Model file for the job. Use its own axes, mm. Face numbers are marked on the shaded views. A direction names the side the tool comes from. Give positions to 0.01 mm unless a question says otherwise; leave off trailing zeros. Loops run counter-clockwise (first coordinate to the right, second up) from the corner with the lowest first, then second, coordinate; pieces in that order, holes last. Notation, with made-up numbers: M -23,-33.5 L 8,-33.5 A12 ccw 8,-10.5 Z; hole C 42,46.25 d3. An arc over 180 degrees is marked long. Answer in a Markdown table with one row per item.
```python
from build123d import *

# Parameters (mm, degrees)
F1_DEPTH = 2.5
F3_DEPTH = 1
F4_DEPTH = 2.5
F5_R     = 5
F6_DEPTH = 2.5


with BuildPart() as f1:
    # F0 (on Top) → F1 (new body)
    with BuildSketch(Plane.XY):
        Polygon((24.5, 28.75), (-24.5, 28.75), (-38, 16), (0, -28), (38, 16), align=None)
    extrude(amount=F1_DEPTH)

    # F2 (on face) → F3 (join)
    with BuildSketch(Plane.XY.offset(2.5)):
        Polygon((-24.5, 28.75), (-38, 16), (0, -28), (38, 16), (24.5, 28.75), align=None)
        Polygon((0, -24.9401175045), (-35.2360005395, 15.8594620676), (-23.7048427287, 26.75), (23.7048427287, 26.75), (35.2360005395, 15.8594620676), align=None, mode=Mode.SUBTRACT)
        with BuildLine():
            Line((22.7133916393, 4.6985002576), (32.2128970418, 15.6979275658))
            Line((32.2128970418, 15.6979275658), (24.9667909899, 22.5414721704))
            Line((24.9667909899, 22.5414721704), (24.9667909899, 15.1083281487))
            Line((24.9667909899, 15.1083281487), (13.8348590806, 15.1083281487))
            ThreePointArc((13.8348590806, 15.1083281487), (13.3444397283, 17.5599116804), (11.9486611802, 19.6341766584))
            ThreePointArc((11.9486611802, 19.6341766584), (8.2805304238, 22.6022293507), (3.7511971493, 23.9249765365))
            ThreePointArc((3.7511971493, 23.9249765365), (-2.3107858295, 24.1330407686), (-8.3545236117, 23.6190738634))
            ThreePointArc((-8.3545236117, 23.6190738634), (-11.0235311437, 22.7778125064), (-13.4403547272, 21.3670376688))
            ThreePointArc((-13.4403547272, 21.3670376688), (-15.212702444, 18.8538109385), (-14.9003509432, 15.7944055113))
            ThreePointArc((-14.9003509432, 15.7944055113), (-11.7357211664, 13.4067953643), (-7.8630894423, 12.5592770055))
            Line((-7.8630894423, 12.5592770055), (8.745636791, 12.5592770055))
            ThreePointArc((8.745636791, 12.5592770055), (12.9047041932, 12.0930390125), (16.8573021999, 10.7174705771))
            ThreePointArc((16.8573021999, 10.7174705771), (20.4582682574, 8.3626966604), (22.7133916393, 4.6985002576))
        make_face()
        with BuildLine():
            Line((25.9667909899, 14.1083281487), (25.9667909899, 20.2215367922))
            Line((25.9667909899, 20.2215367922), (30.8308973116, 15.6276585996))
            Line((30.8308973116, 15.6276585996), (22.9958176649, 6.5554611139))
            ThreePointArc((22.9958176649, 6.5554611139), (20.586748465, 9.6210283517), (17.2501383205, 11.6380433846))
            ThreePointArc((17.2501383205, 11.6380433846), (13.1050428541, 13.0729920976), (8.745636791, 13.5592770055))
            Line((8.745636791, 13.5592770055), (-7.8630894423, 13.5592770055))
            ThreePointArc((-7.8630894423, 13.5592770055), (-11.026529119, 14.1881083225), (-13.7089760974, 15.9789901227))
            ThreePointArc((-13.7089760974, 15.9789901227), (-14.2725466885, 18.498722854), (-12.8559581935, 20.6574127078))
            ThreePointArc((-12.8559581935, 20.6574127078), (-9.8904154712, 22.2976951419), (-6.5607260913, 22.9286774993))
            ThreePointArc((-6.5607260913, 22.9286774993), (-1.4477418736, 23.1604030388), (3.6652423441, 22.9286774993))
            ThreePointArc((3.6652423441, 22.9286774993), (7.8388006263, 21.704705466), (11.2106185406, 18.9574267715))
            ThreePointArc((11.2106185406, 18.9574267715), (12.4121725039, 17.1972104778), (12.8348590806, 15.1083281487))
            Line((12.8348590806, 15.1083281487), (12.8348590806, 14.1083281487))
            Line((12.8348590806, 14.1083281487), (25.9667909899, 14.1083281487))
        make_face(mode=Mode.SUBTRACT)
        with BuildLine():
            ThreePointArc((-6.7919120193, 2.210722072), (-14.655775713, 2.8051401774), (-22.3894476737, 4.349161901))
            Line((-22.3894476737, 4.349161901), (-14.7787371056, -4.4632398095))
            ThreePointArc((-14.7787371056, -4.4632398095), (-7.466030983, -2.8237135208), (-1.0576881468, -6.709181238))
            Line((-1.0576881468, -6.709181238), (7.7347876504, -6.709181238))
            ThreePointArc((7.7347876504, -6.709181238), (9.4624521238, -6.5873541357), (11.1559238285, -6.2242839485))
            ThreePointArc((11.1559238285, -6.2242839485), (13.2256284307, -5.3326624688), (14.9340350181, -3.8629642222))
            ThreePointArc((14.9340350181, -3.8629642222), (15.5006827522, -2.59072721), (15.3472675011, -1.2064799666))
            ThreePointArc((15.3472675011, -1.2064799666), (14.6061136564, -0.1669001783), (13.4981097654, 0.4674203519))
            ThreePointArc((13.4981097654, 0.4674203519), (11.8530830846, 1.0796158365), (10.1323601002, 1.4260382698))
            ThreePointArc((10.1323601002, 1.4260382698), (6.1429657723, 1.8869809032), (2.1316759441, 2.0800848343))
            Line((2.1316759441, 2.0800848343), (-6.7919120193, 2.210722072))
        make_face()
        with BuildLine():
            Line((-14.5836983502, -3.1591329101), (-19.6073624646, 2.6577413276))
            ThreePointArc((-19.6073624646, 2.6577413276), (-13.2424037369, 1.6206816287), (-6.8065499924, 1.2108292129))
            Line((-6.8065499924, 1.2108292129), (2.1170379709, 1.0801919752))
            ThreePointArc((2.1170379709, 1.0801919752), (6.0614887398, 0.8903056837), (9.9844088472, 0.4370436152))
            ThreePointArc((9.9844088472, 0.4370436152), (11.5520586297, 0.255045089), (13.0727859214, -0.1669001783))
            ThreePointArc((13.0727859214, -0.1669001783), (13.8649438936, -0.7048016123), (14.3747050315, -1.5153543791))
            ThreePointArc((14.3747050315, -1.5153543791), (14.560516724, -2.4704828367), (14.1075737774, -3.3316675108))
            ThreePointArc((14.1075737774, -3.3316675108), (12.5743410862, -4.4628960627), (10.8017250896, -5.16169006))
            ThreePointArc((10.8017250896, -5.16169006), (9.2924984584, -5.5712350402), (7.7347876504, -5.709181238))
            Line((7.7347876504, -5.709181238), (-0.5720290784, -5.709181238))
            ThreePointArc((-0.5720290784, -5.709181238), (-7.1112455745, -1.8702452534), (-14.5836983502, -3.1591329101))
        make_face(mode=Mode.SUBTRACT)
        with BuildLine():
            ThreePointArc((9.6052747881, -10.4793192543), (-0.2005916003, -11.6422682343), (-9.9472034322, -10.0576472208))
            Line((-9.9472034322, -10.0576472208), (0.0111213288, -21.5883390493))
            Line((0.0111213288, -21.5883390493), (9.6052747881, -10.4793192543))
        make_face()
        with BuildLine():
            Line((0.0111213288, -20.0583978016), (-7.0874587678, -11.8389892686))
            ThreePointArc((-7.0874587678, -11.8389892686), (-0.1135902043, -12.6442154046), (6.8853861251, -12.0987227742))
            Line((6.8853861251, -12.0987227742), (0.0111213288, -20.0583978016))
        make_face(mode=Mode.SUBTRACT)
        with BuildLine():
            Line((-22.5385466175, 24.7468773517), (-32.1588185263, 15.6610649934))
            Line((-32.1588185263, 15.6610649934), (-26.8728109728, 9.5404246683))
            ThreePointArc((-26.8728109728, 9.5404246683), (-23.2437339896, 18.1532901464), (-16.6198182851, 24.7468773517))
            Line((-16.6198182851, 24.7468773517), (-22.5385466175, 24.7468773517))
        make_face()
        with BuildLine():
            Line((-27.3773424364, 11.6545602424), (-30.7768187961, 15.5907960272))
            Line((-30.7768187961, 15.5907960272), (-22.1409679819, 23.7468773517))
            Line((-22.1409679819, 23.7468773517), (-19.5902141433, 23.7468773517))
            ThreePointArc((-19.5902141433, 23.7468773517), (-24.3653920595, 18.2684544483), (-27.3773424364, 11.6545602424))
        make_face(mode=Mode.SUBTRACT)
        with BuildLine():
            Line((17.1290766448, 24.7468773517), (11.0983193584, 24.7468773517))
            ThreePointArc((11.0983193584, 24.7468773517), (13.4752527233, 22.6732988786), (15.2575302327, 20.0707949334))
            Line((15.2575302327, 20.0707949334), (17.1290766448, 22.5761607289))
            Line((17.1290766448, 22.5761607289), (17.1290766448, 24.7468773517))
        make_face()
        with BuildLine():
            Line((16.1290766448, 22.9084316287), (15.3555178299, 21.8728987756))
            ThreePointArc((15.3555178299, 21.8728987756), (14.6412526921, 22.843669283), (13.8432644406, 23.7468773517))
            Line((13.8432644406, 23.7468773517), (16.1290766448, 23.7468773517))
            Line((16.1290766448, 23.7468773517), (16.1290766448, 22.9084316287))
        make_face(mode=Mode.SUBTRACT)
    extrude(amount=F3_DEPTH)

    # F4 (cut): faces of the model
    f4_faces = [f1.faces().sort_by_distance(p)[0] for p in [
        (5.2313020526, 16.7100656125, 2.5),
        (15.2310227717, 23.0949791253, 2.5),
        (-25.9928017911, 17.89640638, 2.5),
        (-0.20025716, -1.5946330551, 2.5),
        (-0.0583233398, -14.9701076081, 2.5),
    ]]
    extrude(f4_faces, amount=-F4_DEPTH, mode=Mode.SUBTRACT)

    # F5 (on Top) → F6 (join)
    with BuildSketch(Plane.XY):
        Circle(F5_R)
    extrude(amount=-F6_DEPTH)


solid = f1.part
```
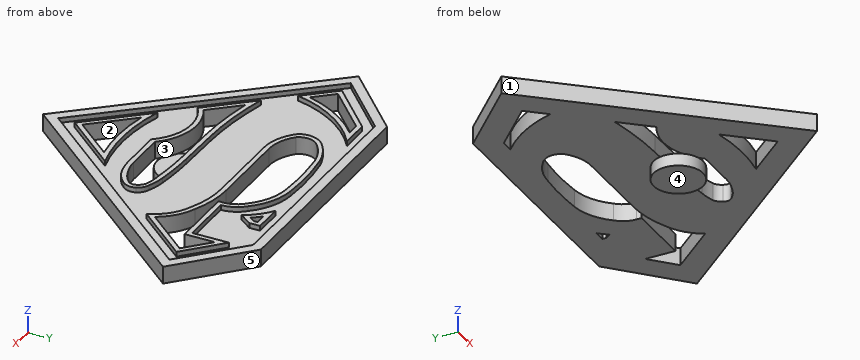
(1) Wall check: L1, parallel to X at y = 22, z = 1.5; L2, parallel to Z at x = 4, y = -1; L3, parallel to Y at x = 21, z = 0.9. Give the ranges that are in metal, low to high.
Established:
| item | result |
|---|---|
| L1 | x = -31.65 to -23.99, -21.43 to -10.63, 7.23 to 15.27, 15.45 to 31.65 |
| L2 | z = -2.5 to 0 |
| L3 | y = -3.68 to 9.24, 14.11 to 28.75 |
(2) Saw through at C-C, the plane x = 20. Give the cut face in (y, z).
Established:
| item | result |
|---|---|
| outline | M -4.84,0 L 10.1,0 L 10.1,3.5 L 8.8,3.5 L 8.8,2.5 L -1.78,2.5 L -1.78,3.5 L -4.84,3.5 Z; M 14.11,0 L 28.75,0 L 28.75,3.5 L 26.75,3.5 L 26.75,2.5 L 15.11,2.5 L 15.11,3.5 L 14.11,3.5 Z |
(3) Mould opens along Y. For the marked faces 3, 4 and 5 say: pulls with the +Y half, pulls with the -Y half, needs draft (parallel to the pull), parting line crosses it, or undercut.
Established:
| item | result |
|---|---|
| face 3 | undercut |
| face 4 | needs draft |
| face 5 | pulls with the +Y half |
(4) Saw through at B-B, the plane x = -11.5. Give the cut face in (y, z), and give its area (3 significant figures).
Established:
| item | result |
|---|---|
| outline | M -14.68,0 L -1.96,0 L -1.96,3.5 L -2.99,3.5 L -2.99,2.5 L -11.62,2.5 L -11.62,3.5 L -14.68,3.5 Z; M 1.45,0 L 14.4,0 L 14.4,3.5 L 13.3,3.5 L 13.3,2.5 L 2.45,2.5 L 2.45,3.5 L 1.45,3.5 Z; M 21.56,0 L 28.75,0 L 28.75,3.5 L 26.75,3.5 L 26.75,2.5 L 22.55,2.5 L 22.55,3.5 L 21.56,3.5 Z |
| area | 91.4 mm2 |
(5) Saw through at A-A, the plane y = 18. Count the separate pieces of the cut face and the enclosed holes in it, and give its area (3 significant figures).
Established:
| item | result |
|---|---|
| separate pieces | 4 |
| enclosed holes | 0 |
| area | 112 mm2 |
(6) Which spindle directions (+Z, -Z, +X, -X, +Y, -Y) get a long thin tool onto all of the face, cutting with end or side? Do the marked faces 1 and 2. Say none if no direction does.
Established:
| item | result |
|---|---|
| face 1 | +Z, -Z, -X, -Y |
| face 2 | +Z, -Z |
(7) Flat gauge pins, fed straight in: P1, Ø8, axis at x = 21.5, y = 20.5, coming from the +Z side; P2, Ø3, axis at x = 0.5, y = -1, coming from the +Z side; P3, Ø1.8, axis at x = 15, z = 2, coming from the -Y side; P4, Ø8, axis at x = 6, y = -9, coming from the -Z side. Where does each tip first touch, or does it go through?
Established:
| item | result |
|---|---|
| P1 | stops at z = 3.5 |
| P2 | stops at z = 0 |
| P3 | stops at y = -11.67 |
| P4 | stops at z = 0 |
